```python
from build123d import *
from build123d.topology import SkipClean

# Parameters (mm, degrees)
BOSS_EXTRUDE1_DEPTH     = 6.35
FILLET1_R               = 12.7
BOSS_EXTRUDE2_DEPTH     = 6.35
FILLET2_R               = 12.7
CUT_EXTRUDE1_DEPTH      = 88.298066989
CUT_EXTRUDE1_DEPTH_BACK = 88.298066989
SKETCH3_R               = 3.96875
FILLET3_R               = 12.7
BOSS_EXTRUDE3_START     = 152.4
BOSS_EXTRUDE3_DEPTH     = 152.4
FILLET4_R               = 12.7
CUT_EXTRUDE2_DEPTH      = 192.450130582
CUT_EXTRUDE2_DEPTH_BACK = 192.450130582
SKETCH5_R               = 3


# Some blends are built 0.0001 mm under size
with BuildPart() as part:
    # Sketch1 → Boss-Extrude1 (new body)
    with BuildSketch(Plane(origin=(0, 0, 0), x_dir=(0, 0, -1), z_dir=(1, 0, 0))):
        Polygon((0, 14.692048969), (50.8, -6.35), (-25.4, -6.35), (-25.4, 6.35), (-25.4, 19.05), (0, 19.05), align=None)
    extrude(amount=BOSS_EXTRUDE1_DEPTH)

    # Fillet1
    # the kernel refuses this fillet: 12.7 mm, written as the material it adds along each edge
    with BuildSketch(Plane(origin=(0, 14.692048969, 0), x_dir=(0, -0.38268343236508373, -0.9238795325112893), z_dir=(1, 0, 0))) as fillet1_piece_1:
        with BuildLine():
            CenterArc((7.608898544, 12.7), FILLET1_R, 223.076533416, 46.923466584)
            Line((-1.667715659, 4.026221762), (-1.853247943, 3.852746197))
            ThreePointArc((-1.853247943, 3.852746197), (-1.068523231, 1.915909289), (-0.234665401, -0.097201592))
            Line((-0.234665401, -0.097201592), (0, -0.254))
            Line((0, -0.254), (7.608898544, -0.254))
            Line((7.608898544, -0.254), (7.608898544, 0))
        make_face()
    extrude(amount=6.35)

    # Sketch2 → Boss-Extrude2 (add)
    with SkipClean():  # the faces are left unmerged after this step: merging them gives an invalid solid
        with BuildSketch(Plane(origin=(6.35, 0, 0), x_dir=(0, 0, -1), z_dir=(1, 0, 0))):
            with BuildLine():
                Line((0, 19.05), (0, 69.85))
                Line((0, 69.85), (-25.4, 69.85))
                Line((-25.4, 69.85), (-25.4, -6.35))
                Line((-25.4, -6.35), (50.8, -6.35))
                Line((50.8, -6.35), (7.02970563, 11.780249557))
                ThreePointArc((7.02970563, 11.780249557), (2.760063939, 14.685258788), (0, 19.05))
            make_face()
        extrude(amount=BOSS_EXTRUDE2_DEPTH)

    # Fillet2
    # the kernel refuses this fillet: 12.7 mm, written as the material it adds along each edge
    with BuildSketch(Plane(origin=(6.35, 19.05, 25.4), x_dir=(-1, 0, 0), z_dir=(0, 0, -1))) as fillet2_piece_1:
        with BuildLine():
            CenterArc((12.7, 10.998522628), FILLET2_R, 180, 60)
            Line((0, 10.998522628), (0, 0))
            Line((0, 0), (6.35, 0))
        make_face()
    extrude(amount=25.4)

    # Sketch3 → Cut-Extrude1 (cut, two sides: drawn at the far end of the back side and taken through both)
    with BuildSketch(Plane(origin=(12.7, 0, 0), x_dir=(0, 0, -1), z_dir=(1, 0, 0)).offset(-CUT_EXTRUDE1_DEPTH_BACK)):
        with Locations((-12.7, 44.45)):
            Circle(SKETCH3_R)
    extrude(amount=CUT_EXTRUDE1_DEPTH + CUT_EXTRUDE1_DEPTH_BACK, mode=Mode.SUBTRACT)

    # Fillet3
    fillet3_edges = [part.edges().sort_by_distance(p)[0] for p in [
        (9.525, 69.85, 0),
        (9.525, 69.85, 25.4),
    ]]
    fillet(fillet3_edges, radius=FILLET3_R - 0.0001)  # a hair under: the kernel refuses the full size

    # Sketch4 → Boss-Extrude3 (add)
    with BuildSketch(Plane.XY.offset(25.4).offset(BOSS_EXTRUDE3_START)):
        with BuildLine():
            Line((6.35, 30.048522628), (6.35, 31.75))
            Line((6.35, 31.75), (12.7, 31.75))
            Line((12.7, 31.75), (12.7, -6.35))
            Line((12.7, -6.35), (0, -6.35))
            Line((0, -6.35), (0, 19.05))
            ThreePointArc((0, 19.05), (4.648522628, 23.698522628), (6.35, 30.048522628))
        make_face()
    extrude(amount=-BOSS_EXTRUDE3_DEPTH)

    # Fillet4
    fillet4_edges = [part.edges().sort_by_distance(p)[0] for p in [
        (9.525, 31.75, 25.4),
    ]]
    fillet(fillet4_edges, radius=FILLET4_R)

    # Sketch5 → Cut-Extrude2 (cut, two sides: drawn at the far end of the back side and taken through both)
    with SkipClean():  # the faces are left unmerged after this step: merging them gives an invalid solid
        with BuildSketch(Plane.ZY.offset(-CUT_EXTRUDE2_DEPTH_BACK)):
            with Locations((139.7, 12.7)):
                Circle(SKETCH5_R)
        extrude(amount=CUT_EXTRUDE2_DEPTH + CUT_EXTRUDE2_DEPTH_BACK, mode=Mode.SUBTRACT)


solid = part.part
```
Here's how the part is built. I have some questions about the finished solid (model axes, mm). A direction names the side the tool comes from. Coordinates: 2 decimals unless noted, no trailing zeros. Loops run counter-clockwise (first coordinate to the right, second up) from the corner with the lowest first, then second, coordinate; pieces in that order, holes last. Notation, with made-up numbers: (59.5, 49.5) - (114.5, 49.5) arc R24 ccw to (114.5, 76.5) - close; hole circle Ø3 at (-19.5, 28.25). An arc over 180 degrees is marked (long way). Answer as CSV lines item,"result".
Q1. If we section it at B-B, the plane x = 9: Give the number of separate pieces and of enclosed holes in the cut face, and give its area (3 significant figures).
Response:
separate pieces,"1"
enclosed holes,"2"
area,"8,170 mm2"
Q2. If we section it at C-C, the plane z = 102: Write out the boundary of the cut face in (x, y), and give its area (3 significant figures).
Response:
outline,"(0, -6.35) - (12.7, -6.35) - (12.7, 31.75) - (6.35, 31.75) - (6.35, 30.05) arc R12.7 cw to (0, 19.05) - close"
area,"424 mm2"
Q3. For pin 1 (6 mm diameter, centred on x = 9.5, y = 1.5, fed in from -Z); pin 2 (1.5 mm diameter, centred on x = 4, y = 30.5, fed in from +Z); pin 3 (5 mm diameter, centred on x = 10, z = 59, fed in from +Y); pin 4 (6.5 mm diameter, centred on x = 7, y = 33, fed in from -Z), each with a flat end and sliding along its axis, tell me the tip position at first contact or that it passes through.
Response:
pin 1,"z = -39.09"
pin 2,"through"
pin 3,"y = 31.75"
pin 4,"z = 0"
Q4. If we section it at D-D, the plane y = 5.5: Write out the boundary of the cut face in (x, z), and give its area (3 significant figures).
Response:
outline,"(0, -22.19) - (12.7, -22.19) - (12.7, 177.8) - (0, 177.8) - close"
area,"2,540 mm2"
Q5. If I drill on L1, parallel to Y at x = 8.75, z = 12.7; L2, parallel to Y at x = 7.25, z = 139.7; L3, parallel to Y at x = 10.75, z = 97.5, over which ranges is the centre line in solid material (lowest first)? Write a range as [from, to].
Response:
L1,"[-6.35, 40.48], [48.42, 69.85]"
L2,"[-6.35, 9.7], [15.7, 31.75]"
L3,"[-6.35, 31.75]"
Q6. If we section it at A-A, the plane z = 139.7: Write out the boundary of the cut face in (x, y).
Response:
outline,"(0, -6.35) - (12.7, -6.35) - (12.7, 9.7) - (0, 9.7) - close; (0, 15.7) - (12.7, 15.7) - (12.7, 31.75) - (6.35, 31.75) - (6.35, 30.05) arc R12.7 cw to (0, 19.05) - close"
Q7. For faces 5 (the face through (6.35, 45, 23)), 6 (the face through (12.7, 15, 65)), 7 (the face through (9, 51, 25.4)), which set-ups out of +Z, -Z, +X, -X, +Y, -Y let a thin tool reach every point of the face, with its end or its side?
Response:
face 5,"+Z, -Z, -X, +Y"
face 6,"+Z, -Z, +X, +Y, -Y"
face 7,"+Z, +X, -X, +Y"
Q8. We'd pull the mould along Z, two halves only. Please class faces 1 (the face through (9, 38, 0)), 2 (the face through (9.48, 47.8, 10.57)), 3 (the face through (9.57, 35.37, 29.22)), 4 (the face through (6.44, 13.6, 142.56)): pulls with the +Z half, pulls with the -Z half, needs draft (parallel to the pull), parting line crosses it, or undercut.
Response:
face 1,"pulls with the -Z half"
face 2,"undercut"
face 3,"pulls with the +Z half"
face 4,"undercut"
